from build123d import *

# Parameters (mm, degrees)
SKETCH1_W           = 12.7
SKETCH1_H           = 88.9
SKETCH1_W_2         = 4.62
SKETCH1_H_2         = 4.62
BOSS_EXTRUDE1_DEPTH = 1.5875
BOSS_EXTRUDE2_DEPTH = 1.5875


with BuildPart() as part:
    # Sketch1 → Boss-Extrude1 (new body)
    with BuildSketch(Plane(origin=(0, 0, 0), x_dir=(1, 0, 0), z_dir=(0, 1, 0))):
        with Locations((6.358064201, 57.44278115)):
            Rectangle(SKETCH1_W, SKETCH1_H)
        with Locations((6.358064201, 95.54278115)):
            Rectangle(SKETCH1_W_2, SKETCH1_H_2, mode=Mode.SUBTRACT)
        with Locations((6.358064201, 31.89278115)):
            Rectangle(SKETCH1_W_2, SKETCH1_H_2, mode=Mode.SUBTRACT)
    extrude(amount=BOSS_EXTRUDE1_DEPTH)

    # Sketch2 → Boss-Extrude2 (add)
    with BuildSketch(Plane.XZ):
        Polygon((0.008064201, -20.068103044), (0.008064201, -15.232133805), (-85.280307223, -30.270774828), (-84.453307777, -34.960921752), align=None)
    extrude(amount=-BOSS_EXTRUDE2_DEPTH)


solid = part.part
Could you check a few things on this model? Use its own coordinates, in mm. Give positions to 0.01 mm unless a question says otherwise; leave off trailing zeros. Write each loop counter-clockwise with the first axis right and the second up, starting at its lowest first coordinate (ties: lowest second). Pieces come first, ordered by that corner, then holes. Notation, with made-up numbers: (73, -23) -> (127, -23) arc R25 ccw to (127, -7) -> close; hole circle Ø10 at (-29, 44.5). An arc over 180 degrees is marked (long way). Answer as a JSON object with one key per item and string values.
Q1. Suppose I cut it at D-D on x = -59.5. Write out the boundary of the cut face in (y, z).
Taken from the geometry:
{"outline": "(0, -30.56) -> (1.59, -30.56) -> (1.59, -25.73) -> (0, -25.73) -> close"}
Q2. Suppose I cut it at A-A on y = 1. Write out the boundary of the cut face in (x, z), then the cut area to 3 significant figures.
Taken from the geometry:
{"outline": "(-85.28, -30.27) -> (-84.45, -34.96) -> (0.01, -20.07) -> (0.01, -101.89) -> (12.71, -101.89) -> (12.71, -12.99) -> (0.01, -12.99) -> (0.01, -15.23) -> close; hole (4.05, -97.85) -> (8.67, -97.85) -> (8.67, -93.23) -> (4.05, -93.23) -> close; hole (4.05, -34.2) -> (8.67, -34.2) -> (8.67, -29.58) -> (4.05, -29.58) -> close", "area": "1,500 mm²"}
Q3. We'd pull the mould along X, two halves only. Please class faces 1 (the flat face through (-42.039, 0.783, -22.646)), 2 (the flat face through (3, 0, -48)), 3 (the flat face through (-42.81, 0.78, -27.62)): released by +X, released by -X, zero draft, split by the parting line, or undercut.
Taken from the geometry:
{"face 1": "released by -X", "face 2": "zero draft", "face 3": "undercut"}
Q4. Suppose I cut it at C-C on z = -83.5. Write out the boundary of the cut face in (x, y).
Taken from the geometry:
{"outline": "(0.01, 0) -> (12.71, 0) -> (12.71, 1.59) -> (0.01, 1.59) -> close"}
Q5. Will this pin go through, and if not, where does the flat tip stop? pin 1 Ø0.8 at (y, z) = (0.5, -61.5) entering from -X.
Taken from the geometry:
{"pin 1": "stops at x = 0.01"}
Q6. Suppose I cut it at B-B on x = 6. Write out the boundary of the cut face in (y, z).
Taken from the geometry:
{"outline": "(0, -101.89) -> (1.59, -101.89) -> (1.59, -97.85) -> (0, -97.85) -> close; (0, -93.23) -> (1.59, -93.23) -> (1.59, -34.2) -> (0, -34.2) -> close; (0, -29.58) -> (1.59, -29.58) -> (1.59, -12.99) -> (0, -12.99) -> close"}
Q7. Please list where these lines run through material, in increasing order: L1, parallel to Z at x = 5.5, y = 0.7; L2, parallel to X at y = 0.8, z = -95.5; L3, parallel to X at y = 0.8, z = -72.5.
Taken from the geometry:
{"L1": "z = -101.89 to -97.85, -93.23 to -34.2, -29.58 to -12.99", "L2": "x = 0.01 to 4.05, 8.67 to 12.71", "L3": "x = 0.01 to 12.71"}
